Source: CAD feature listing. Evaluate the final solid. Frame: model axes, mm. A direction names the side the tool comes from. Give positions to 0.01 mm unless a question says otherwise; leave off trailing zeros. Order: outer loops, then holes, each group sorted by start corner. A loop starts at its lowest first (then second) coordinate and runs counter-clockwise, first axis right, second up. Notation, with made-up numbers: M 42.25,40 L 72.25,40 A20 cw 72.25,66 Z; hole C 73,-36.5 d4. An arc over 180 degrees is marked long. Use CSV: the item, a comma, the result in double quotes. Start each with the question number.
1. Section query C-C, the plane x = -6. Return the cut outline in (y, z).
2. Pin query (flat end, axial travel): P1, Ø3.5, axis at x = 28, z = 215.3, coming from the -Y side; P2, Ø1, axis at x = -122, y = 5.5, coming from the -Z side; P3, Ø6.5, axis at x = -132, y = 4.5, coming from the -Z side; P4, Ø4, axis at x = -132, y = 6, coming from the -Z side. Return the tip coordinate at first contact, or that it passes through.
3. Section query B-B, the plane z = 168.25. Return the cut outline in (x, y).
4. Section query D-D, the plane y = 5. State how many separate pieces and enclosed holes the cut face has, plus the area to 3 significant figures.
5. Reachability of faces 1 (the cylindrical face through (2.67, 6.26, -265.74)), 2 (the cylindrical face through (121.02, 6.26, 168.39)) from +Z, -Z, +X, -X, +Y, -Y: full face, straight path, thin tool, end or side. Return the list, or none.
6. Section query A-A, the plane z = -168.25. Return the cut outline in (x, y).
7. Line query: line 1 along X through (y, z) = (3.25, 101); line 2 along X through (y, z) = (4, 152.4); line 3 along Z through (x, y) = (6, 7.75). Output: solid intervals per line, ascending. Write a range as [from, to].
8. Mould query, pull axis X, two halves, no side actions, for faces 3 (the flat face through (175, 6, 3)), 4 (the flat face through (-175, 6, -3)), 5 (the flat face through (-134, 6, -174.6)). Classes: released by +X, released by -X, zero draft, split by the parting line, or undercut.
from build123d import *

# Parameters (mm, degrees)
SKETCH1_R           = 1.5
SKETCH1_R_2         = 3.5687
BOSS_EXTRUDE1_DEPTH = 12.7


with BuildPart() as part:
    # Sketch1 → Boss-Extrude1 (new body)
    with BuildSketch(Plane(origin=(0, 0, 0), x_dir=(1, 0, 0), z_dir=(0, 1, 0))):
        with BuildLine():
            Line((175, -200), (175, 200))
            ThreePointArc((175, 200), (0, 265.753645318), (-175, 200))
            Line((-175, 200), (-175, -200))
            ThreePointArc((-175, -200), (0, -265.753645318), (175, -200))
        make_face()
        with Locations((20, -145.3)):
            Circle(SKETCH1_R, mode=Mode.SUBTRACT)
        with Locations((-20, -145.3)):
            Circle(SKETCH1_R, mode=Mode.SUBTRACT)
        with Locations((28, -215.3)):
            Circle(SKETCH1_R, mode=Mode.SUBTRACT)
        with Locations((-28, -215.3)):
            Circle(SKETCH1_R, mode=Mode.SUBTRACT)
        with Locations((-159.12, -101.6)):
            Circle(SKETCH1_R_2, mode=Mode.SUBTRACT)
        with Locations((-159.12, -152.4)):
            Circle(SKETCH1_R_2, mode=Mode.SUBTRACT)
        with Locations((-159.12, 152.4)):
            Circle(SKETCH1_R_2, mode=Mode.SUBTRACT)
        with Locations((-159.12, 101.6)):
            Circle(SKETCH1_R_2, mode=Mode.SUBTRACT)
        with Locations((159.12, -152.4)):
            Circle(SKETCH1_R_2, mode=Mode.SUBTRACT)
        with Locations((159.12, -101.6)):
            Circle(SKETCH1_R_2, mode=Mode.SUBTRACT)
        with Locations((159.12, 101.6)):
            Circle(SKETCH1_R_2, mode=Mode.SUBTRACT)
        with Locations((159.12, 152.4)):
            Circle(SKETCH1_R_2, mode=Mode.SUBTRACT)
        with BuildLine():
            Line((-12.7, -161.9), (12.7, -161.9))
            ThreePointArc((12.7, -161.9), (19.05, -168.25), (12.7, -174.6))
            Line((12.7, -174.6), (-12.7, -174.6))
            ThreePointArc((-12.7, -174.6), (-19.05, -168.25), (-12.7, -161.9))
        make_face(mode=Mode.SUBTRACT)
        with BuildLine():
            Line((-140.07, -161.9), (-127.37, -161.9))
            ThreePointArc((-127.37, -161.9), (-121.02, -168.25), (-127.37, -174.6))
            Line((-127.37, -174.6), (-140.07, -174.6))
            ThreePointArc((-140.07, -174.6), (-146.42, -168.25), (-140.07, -161.9))
        make_face(mode=Mode.SUBTRACT)
        with BuildLine():
            Line((127.37, -161.9), (140.07, -161.9))
            ThreePointArc((140.07, -161.9), (146.42, -168.25), (140.07, -174.6))
            Line((140.07, -174.6), (127.37, -174.6))
            ThreePointArc((127.37, -174.6), (121.02, -168.25), (127.37, -161.9))
        make_face(mode=Mode.SUBTRACT)
        with BuildLine():
            Line((-140.07, 174.6), (-127.37, 174.6))
            ThreePointArc((-127.37, 174.6), (-121.02, 168.25), (-127.37, 161.9))
            Line((-127.37, 161.9), (-140.07, 161.9))
            ThreePointArc((-140.07, 161.9), (-146.42, 168.25), (-140.07, 174.6))
        make_face(mode=Mode.SUBTRACT)
        with BuildLine():
            Line((127.37, 174.6), (140.07, 174.6))
            ThreePointArc((140.07, 174.6), (146.42, 168.25), (140.07, 161.9))
            Line((140.07, 161.9), (127.37, 161.9))
            ThreePointArc((127.37, 161.9), (121.02, 168.25), (127.37, 174.6))
        make_face(mode=Mode.SUBTRACT)
        with BuildLine():
            Line((-12.7, 25.4), (12.7, 25.4))
            ThreePointArc((12.7, 25.4), (19.05, 19.05), (12.7, 12.7))
            Line((12.7, 12.7), (-12.7, 12.7))
            ThreePointArc((-12.7, 12.7), (-19.05, 19.05), (-12.7, 25.4))
        make_face(mode=Mode.SUBTRACT)
    extrude(amount=BOSS_EXTRUDE1_DEPTH)


solid = part.part
Result set:
1,outline,"M 0,-265.69 L 12.7,-265.69 L 12.7,-25.4 L 0,-25.4 Z; M 0,-12.7 L 12.7,-12.7 L 12.7,161.9 L 0,161.9 Z; M 0,174.6 L 12.7,174.6 L 12.7,265.69 L 0,265.69 Z"
2,P1,"y = 0"
2,P2,"z = -236.35"
2,P3,"z = -232.48"
2,P4,"z = -231.79"
3,outline,"M -175,0 L -146.42,0 L -146.42,12.7 L -175,12.7 Z; M -121.02,0 L -19.05,0 L -19.05,12.7 L -121.02,12.7 Z; M 19.05,0 L 121.02,0 L 121.02,12.7 L 19.05,12.7 Z; M 146.42,0 L 175,0 L 175,12.7 L 146.42,12.7 Z"
4,separate pieces,"1"
4,enclosed holes,"18"
4,area,"169,000 mm2"
5,face 1,"-Z, +Y, -Y"
5,face 2,"+Y, -Y"
6,outline,"M -175,0 L -146.42,0 L -146.42,12.7 L -175,12.7 Z; M -121.02,0 L 121.02,0 L 121.02,12.7 L -121.02,12.7 Z; M 146.42,0 L 175,0 L 175,12.7 L 146.42,12.7 Z"
7,line 1,"[-175, -162.64], [-155.6, 155.6], [162.64, 175]"
7,line 2,"[-175, -162.69], [-155.55, 155.55], [162.69, 175]"
7,line 3,"[-265.69, -25.4], [-12.7, 161.9], [174.6, 265.69]"
8,face 3,"released by +X"
8,face 4,"released by -X"
8,face 5,"undercut"
